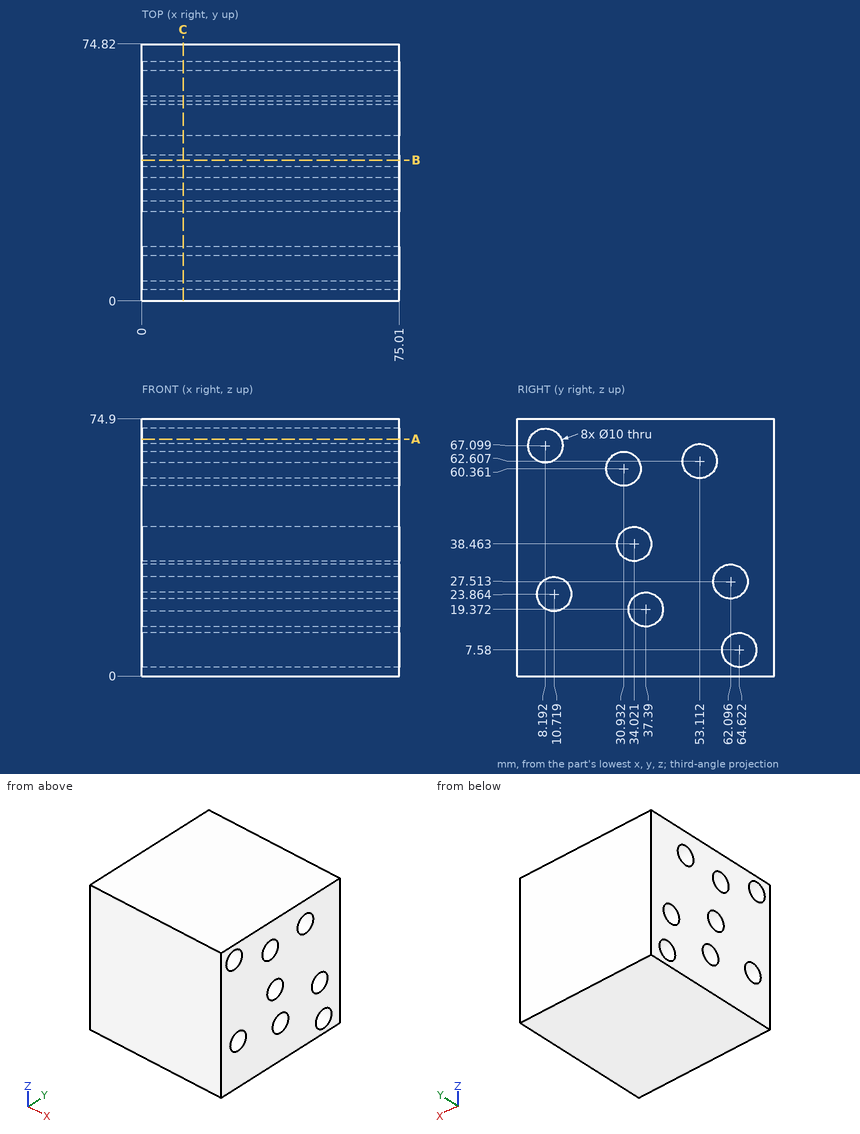
Check sheet for the drawn part. Datum: minimum x, y, z corner. Units: mm. Give positions to 0.01 mm unless a question says otherwise; leave off trailing zeros. Write each loop counter-clockwise with the first axis right and the second up, starting at its lowest first coordinate (ties: lowest second). Pieces come first, ordered by that corner, then holes.
(1) Material ranges on line 1 (Z direction, x = 54.5, y = 62) (1 decimal); line 2 (Z direction, x = 51, y = 12) (1 decimal); line 3 (Y direction, x = 40.5, z = 64.5) (1 decimal), recorded low to high.
(2) Gauge pin test, flat ends, axial feed: pin 1 (1.5 mm diameter, centred on x = 57, y = 48.5, fed in from -Z); pin 2 (9 mm diameter, centred on y = 62.1, z = 27.51, fed in from -X). Record the tip position at first contact, or that the pin passes through.
(3) Cross-section at C-C (x = 12). State how many separate pieces and enclosed holes the cut face has, plus the area to 3 significant figures.
(4) Cross-section at B-B (y = 41). Enter the section's corners in (x, z), plus the area to 3 significant figures.
(5) Cross-section at A-A (z = 69). Enter the section's corners in (x, y), plus the area to 3 significant figures.
Worked out:
1. line 1: z = 0 to 3.3, 11.8 to 22.5, 32.5 to 74.9
1. line 2: z = 0 to 19, 28.7 to 63.9, 70.3 to 74.9
1. line 3: y = 0 to 3.9, 12.5 to 28.1, 33.7 to 48.5, 57.7 to 74.8
2. pin 1: stops at z = 0
2. pin 2: passes through
3. separate pieces: 1
3. enclosed holes: 8
3. area: 4,980 mm2
4. outline: (0, 0) - (75.01, 0) - (75.01, 15.91) - (0, 15.91) - close; (0, 22.83) - (75.01, 22.83) - (75.01, 74.9) - (0, 74.9) - close
4. area: 5,100 mm2
5. outline: (0, 0) - (75.01, 0) - (75.01, 3.57) - (0, 3.57) - close; (0, 12.82) - (75.01, 12.82) - (75.01, 74.82) - (0, 74.82) - close
5. area: 4,920 mm2
